Input: part model. Units: mm. Frame: model coordinates. A direction names the side the tool comes from. Coordinates: 2 decimals unless noted, no trailing zeros. Loops run counter-clockwise (first coordinate to the right, second up) from the corner with the lowest first, then second, coordinate; pieces in that order, holes last.
```python
from build123d import *

# Parameters (mm, degrees)
PAD_DEPTH       = 6
POCKET_DEPTH    = 3
SKETCH002_W     = 18.4
SKETCH002_H     = 20.85
POCKET001_DEPTH = 3
SKETCH003_W     = 8
SKETCH003_H     = 1.65
POCKET002_DEPTH = 3
PAD001_DEPTH    = 3
SKETCH005_W     = 193
SKETCH005_H     = 5.95
PAD002_DEPTH    = 3


with BuildPart() as part:
    # Sketch → Pad (new body)
    with BuildSketch(Plane.XY):
        with BuildLine():
            ThreePointArc((-95, 37.5), (-132.5, 0), (-95, -37.5))
            Line((-95, -37.5), (95, -37.5))
            ThreePointArc((95, -37.5), (132.5, 0), (95, 37.5))
            Line((-95, 37.5), (95, 37.5))
        make_face()
    extrude(amount=PAD_DEPTH)

    # Sketch001 (on Face6 of Pad) → Pocket (cut)
    with BuildSketch(Plane.XY.offset(6)):
        with BuildLine():
            ThreePointArc((-98.5, 6), (-104.5, 0), (-98.5, -6))
            Line((-98.5, -6), (98.5, -6))
            ThreePointArc((98.5, -6), (104.5, 0), (98.5, 6))
            Line((-98.5, 6), (98.5, 6))
        make_face()
    extrude(amount=-POCKET_DEPTH, mode=Mode.SUBTRACT)

    # Sketch002 (on Face5 of Pocket) → Pocket001 (cut)
    with BuildSketch(Plane.XY.offset(6)):
        with Locations((0, -25.425)):
            Rectangle(SKETCH002_W, SKETCH002_H)
    extrude(amount=-POCKET001_DEPTH, mode=Mode.SUBTRACT)

    # Sketch003 (on Face5 of Pocket001) → Pocket002 (cut)
    with BuildSketch(Plane.XY.offset(6)):
        with Locations((0, -36.675)):
            Rectangle(SKETCH003_W, SKETCH003_H)
    extrude(amount=-POCKET002_DEPTH, mode=Mode.SUBTRACT)

    # Sketch004 (on Face5 of Pocket002) → Pad001 (join)
    with BuildSketch(Plane.XY.offset(6)):
        with BuildLine():
            ThreePointArc((-95, 37.5), (-132.5, 0), (-95, -37.5))
            Line((-95, -37.5), (95, -37.5))
            ThreePointArc((95, -37.5), (132.5, 0), (95, 37.5))
            Line((-95, 37.5), (95, 37.5))
        make_face()
        with BuildLine():
            ThreePointArc((-98.5, 6), (-104.5, 0), (-98.5, -6))
            Line((-98.5, -6), (98.5, -6))
            ThreePointArc((98.5, -6), (104.5, 0), (98.5, 6))
            Line((-98.5, 6), (98.5, 6))
        make_face(mode=Mode.SUBTRACT)
    extrude(amount=PAD001_DEPTH)

    # Sketch005 (on Face12 of Pad001) → Pad002 (join)
    with BuildSketch(Plane.XY.offset(9)):
        with BuildLine():
            ThreePointArc((-95, 37.5), (-132.5, 0), (-95, -37.5))
            Line((-95, -37.5), (95, -37.5))
            ThreePointArc((95, -37.5), (132.5, 0), (95, 37.5))
            Line((-95, 37.5), (95, 37.5))
        make_face()
        Rectangle(SKETCH005_W, SKETCH005_H, mode=Mode.SUBTRACT)
    extrude(amount=PAD002_DEPTH)


solid = part.part
```
Item 1: Mould query, pull axis X, two halves, no side actions, for faces 1 (the face through (132.49, -0.82, 5.92)), 2 (the face through (-104.5, 0.1, 6)), 3 (the face through (-2, 9, 12)). Classes: +X half, -X half, draft (parallel to the pull), parting line (faces both ways), or undercut.
Result:
face 1: +X half
face 2: undercut
face 3: draft
Item 2: Contact query for flat-ended pins moving along their axis: P1, Ø3.5, axis at y = -30, z = 4, coming from the -X side; P2, Ø2.5, axis at y = -23.5, z = 4, coming from the +X side; P3, Ø0.9, axis at y = -0.5, z = 11, coming from the -X side. Output: stop coordinate, or through.
Result:
P1: stops at x = -119.66
P2: stops at x = 125.19
P3: stops at x = -132.5
Item 3: Section query D-D (x = 115). Output: boundary loops of the cut face in (y, z), then the cut area to 3 significant figures.
Result:
outline: (-31.72, 0) - (31.72, 0) - (31.72, 12) - (-31.72, 12) - close
area: 761 mm2
Item 4: Section query B-B (y = -0.5). Output: boundary loops of the cut face in (x, z), then the cut area to 3 significant figures.
Result:
outline: (-132.5, 0) - (132.5, 0) - (132.5, 12) - (96.5, 12) - (96.5, 9) - (104.48, 9) - (104.48, 3) - (-104.48, 3) - (-104.48, 9) - (-96.5, 9) - (-96.5, 12) - (-132.5, 12) - close
area: 1,350 mm2
Item 5: Line query: L1, parallel to Y at x = -52.5, z = 8.25; L2, parallel to Z at x = -2.5, y = -5; L3, parallel to Z at x = -6.5, y = -29.5. Output: solid intervals per line, ascending.
Result:
L1: y = -37.5 to -6, 6 to 37.5
L2: z = 0 to 3, 9 to 12
L3: z = 0 to 3, 6 to 12
Item 6: Section query A-A (x = 87). Output: boundary loops of the cut face in (y, z) (3 decimals).
Result:
outline: (-37.5, 0) - (37.5, 0) - (37.5, 12) - (2.975, 12) - (2.975, 9) - (6, 9) - (6, 3) - (-6, 3) - (-6, 9) - (-2.975, 9) - (-2.975, 12) - (-37.5, 12) - close
Item 7: Reachability of faces 4 (the face through (-2, 1, 0)), 5 (the face through (104.5, -0.1, 6)) from +Z, -Z, +X, -X, +Y, -Y: full face, straight path, thin tool, end or side. Return the list, or none.
Result:
face 4: -Z, +X, -X, +Y, -Y
face 5: none
Item 8: Section query C-C (y = 29). Output: boundary loops of the cut face in (x, z), then the cut area to 3 significant figures.
Result:
outline: (-118.77, 0) - (118.77, 0) - (118.77, 12) - (-118.77, 12) - close
area: 2,850 mm2
